```python
from build123d import *

# Parameters (mm, degrees)
SKETCH2_R           = 39.788735773
SKETCH2_R_2         = 27.75
BOSS_EXTRUDE1_DEPTH = 12
BOSS_EXTRUDE2_START = 1.5
SKETCH3_R           = 27.75
SKETCH3_R_2         = 3
BOSS_EXTRUDE2_DEPTH = 15


with BuildPart() as part:
    # Sketch1 → Revolve1 (revolve)
    with BuildSketch(Plane.XY):
        Polygon((3, 22), (3, 0), (27.75, 0), (27.75, 12), (15, 12), (15, 22), align=None)
    revolve(axis=Axis((0, 0, 0), (0, 1, 0)))



with BuildPart() as body_2:
    # Sketch2 → Boss-Extrude1 (new body)
    with BuildSketch(Plane.XZ):
        Circle(SKETCH2_R)
        Circle(SKETCH2_R_2, mode=Mode.SUBTRACT)
    extrude(amount=-BOSS_EXTRUDE1_DEPTH)


with BuildPart() as part_1:
    add(part.part)

    add(body_2.part)  # Boss-Extrude2 merges body 2
    # Sketch3 → Boss-Extrude2 (add)
    with BuildSketch(Plane.XZ.offset(BOSS_EXTRUDE2_START)):
        Circle(SKETCH3_R)
        Circle(SKETCH3_R_2, mode=Mode.SUBTRACT)
    extrude(amount=-BOSS_EXTRUDE2_DEPTH)


solid = part_1.part
```
Can you work these out from the model? Positions are in its coordinate system, mm. A direction names the side the tool comes from. Coordinates: 2 decimals unless noted, no trailing zeros. Loops run counter-clockwise (first coordinate to the right, second up) from the corner with the lowest first, then second, coordinate; pieces in that order, holes last. Notation, with made-up numbers: M 69,76 L 75,76 A34 cw 75,106 Z; hole C 79.5,-29 d3. An arc over 180 degrees is marked long. Put each result on its own line as item: value. Start each with the question number.
(1) Imagine slicing it at C-C on x = 9. List the corners of the cut face in (y, z) for me, and give its area (3 significant figures).
(2) Imagine slicing it at D-D on y = 3.5. List the corners of the cut face in (x, z) for me.
(3) Imagine slicing it at B-B on z = 0. List the corners of the cut face in (x, y) for me, and give its area (3 significant figures).
(4) I need wall thicknesses on probe 1 along Z at (x, y) = (0, 16.5); probe 2 along Z at (x, y) = (0, 6). Which ranges of each line are inside material? Lowest first, please.
(5) Will these pins go through, and if not, where does the flat tip stop? pin 1 Ø2 at (x, y) = (-21, 4) entering from +Z; pin 2 Ø1.5 at (y, z) = (8.5, 13) entering from -X; pin 3 Ø5 at (y, z) = (3, -12.5) entering from -X; pin 4 Ø7 at (x, z) = (0, 0) entering from +Y.
(6) Imagine slicing it at A-A on x = 0. List the corners of the cut face in (y, z) for me, and give its area (3 significant figures).
(7) Which directions (+Z, -Z, +X, -X, +Y, -Y) give clear straight access to the entire face, cutting with the end or side of a thin tool? Please do faces 1 (the face through (-27, 0, -8)), 2 (the face through (26.469, 12.74, 8.335)), 3 (the face through (0, -1.5, -6)).
Worked answers:
1. outline: M -1.5,-26.25 L 0,-26.25 L 0,-38.76 L 12,-38.76 L 12,-26.25 L 13.5,-26.25 L 13.5,-12 L 22,-12 L 22,12 L 13.5,12 L 13.5,26.25 L 12,26.25 L 12,38.76 L 0,38.76 L 0,26.25 L -1.5,26.25 Z
1. area: 1,290 mm2
2. outline: C 0,0 d79.58; hole C 0,0 d6
3. outline: M -39.79,0 L -27.75,0 L -27.75,-1.5 L -3,-1.5 L -3,22 L -15,22 L -15,13.5 L -27.75,13.5 L -27.75,12 L -39.79,12 Z; M 3,-1.5 L 27.75,-1.5 L 27.75,0 L 39.79,0 L 39.79,12 L 27.75,12 L 27.75,13.5 L 15,13.5 L 15,22 L 3,22 Z
3. area: 1,240 mm2
4. probe 1: z = -15 to -3, 3 to 15
4. probe 2: z = -39.79 to -3, 3 to 39.79
5. pin 1: stops at z = 34.4
5. pin 2: stops at x = -37.86
5. pin 3: stops at x = -38.51
5. pin 4: stops at y = 22
6. outline: M -1.5,-27.75 L 0,-27.75 L 0,-39.79 L 12,-39.79 L 12,-27.75 L 13.5,-27.75 L 13.5,-15 L 22,-15 L 22,-3 L -1.5,-3 Z; M -1.5,3 L 22,3 L 22,15 L 13.5,15 L 13.5,27.75 L 12,27.75 L 12,39.79 L 0,39.79 L 0,27.75 L -1.5,27.75 Z
6. area: 1,240 mm2
7. face 1: -Y
7. face 2: +Y
7. face 3: +Z, -Z, +X, -X, -Y
